CAD build for the part. Positions are in the model's coordinates, mm. Face numbers are marked on the shaded views. A direction names the side the tool comes from. Coordinates: 2 decimals unless noted, no trailing zeros. Loops run counter-clockwise (first coordinate to the right, second up) from the corner with the lowest first, then second, coordinate; pieces in that order, holes last.
1) Saw through at D-D, the plane x = 17. Write the cut outline in (y, z).
2) Pin check, flat tips, straight feed: pin 1 Ø3 at (y, z) = (13.5, 6) entering from -X; pin 2 Ø2 at (x, z) = (45, 4.5) entering from +Y; pin 3 Ø3 at (y, z) = (-2, 4) entering from -X. Stop position of each tip, or through.
3) Two-plate mould, pull along Y, no slides. Class the marked faces 4, 5 and 6: +Y half, -Y half, draft (parallel to the pull), parting line (faces both ways), or undercut.
4) Saw through at B-B, the plane y = -33. Write the cut outline in (x, z), and give its area (3 significant figures).
5) Saw through at C-C, the plane z = 3.25. Give the number of separate pieces and of enclosed holes in the cut face, and give its area (3 significant figures).
6) Wall check: line 1 along Y through (x, z) = (50, 5.25); line 2 along Y through (x, z) = (-13, 6.25); line 3 along X through (y, z) = (12, 1.75). Give the ranges that are in metal, low to high.
7) Saw through at A-A, the plane x = 45. Write the cut outline in (y, z), and give its area (3 significant figures).
8) Which spindle directions (+Z, -Z, +X, -X, +Y, -Y) get a long thin tool onto all of the face, cutting with end or side? Do the marked faces 1, 2 and 3. Say none if no direction does.
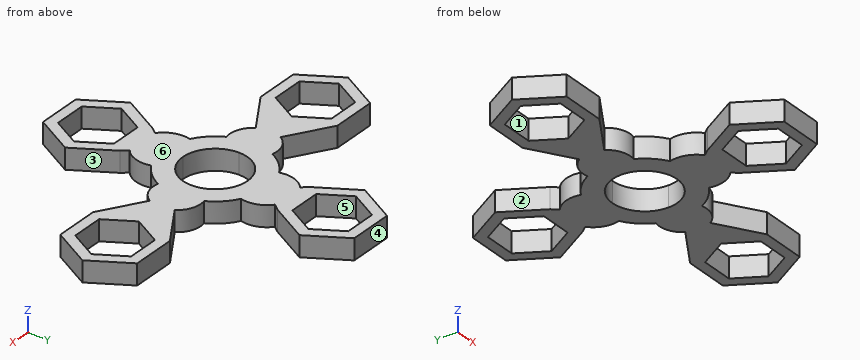
```python
from build123d import *

# Parameters (mm, degrees)
F1_DEPTH = 7


# Not quite as in the source:
# - a feature names something its author has since deleted; it is built from what else it names


with BuildPart() as f1:
    # F0 (on Top) → F1 (new body)
    with BuildSketch(Plane.XY):
        Polygon((-53.4446571767, -12.9903810568), (-38.4446571767, -12.9903810568), (-30.9446571767, 0), (-38.4446571767, 12.9903810568), (-53.4446571767, 12.9903810568), (-60.9446571767, 0), align=None)
        Polygon((-56.8446571767, 0), (-51.3946571767, 9.4396769013), (-40.4946571767, 9.4396769013), (-35.0446571767, 0), (-40.4946571767, -9.4396769013), (-51.3946571767, -9.4396769013), align=None, mode=Mode.SUBTRACT)
        with BuildLine():
            ThreePointArc((0, 10.9), (7.7074639149, 7.7074639149), (10.9, 0))
            Line((10.9, 0), (17.5, 0))
            ThreePointArc((17.5, 0), (17.0367250374, 4), (15.6714285714, 7.78821716))
            ThreePointArc((15.6714285714, 7.78821716), (12.7504247795, 11.9865202599), (8.7403572641, 15.1610077137))
            ThreePointArc((8.7403572641, 15.1610077137), (4.5239565101, 16.9051417473), (0, 17.5))
            Line((0, 17.5), (0, 10.9))
        make_face()
        with BuildLine():
            Line((17.5, 0), (10.9, 0))
            ThreePointArc((10.9, 0), (7.7074639149, -7.7074639149), (0, -10.9))
            Line((0, -10.9), (0, -17.5))
            ThreePointArc((0, -17.5), (4.5925968465, -16.8866235289), (8.8632518819, -15.0894919092))
            ThreePointArc((8.8632518819, -15.0894919092), (12.7990151761, -11.9346223452), (15.6714285714, -7.78821716))
            ThreePointArc((15.6714285714, -7.78821716), (17.0367250374, -4), (17.5, 0))
        make_face()
        with BuildLine():
            ThreePointArc((-10.9, 0), (-7.7074639149, 7.7074639149), (0, 10.9))
            Line((0, 10.9), (0, 17.5))
            ThreePointArc((0, 17.5), (-4.5239565101, 16.9051417473), (-8.7403572641, 15.1610077137))
            ThreePointArc((-8.7403572641, 15.1610077137), (-12.7504247795, 11.9865202599), (-15.6714285714, 7.78821716))
            ThreePointArc((-15.6714285714, 7.78821716), (-17.0367250374, 4), (-17.5, 0))
            Line((-17.5, 0), (-10.9, 0))
        make_face()
        Polygon((-7.5, 26.5479130202), (0, 26.5479130202), (7.5, 26.5479130202), (15, 39.5382940769), (7.5, 52.5286751337), (-7.5, 52.5286751337), (-15, 39.5382940769), align=None)
        Polygon((-10.9, 39.5382940769), (-5.45, 48.9779709782), (5.45, 48.9779709782), (10.9, 39.5382940769), (5.45, 30.0986171757), (-5.45, 30.0986171757), align=None, mode=Mode.SUBTRACT)
        Polygon((30.9, 0), (38.4, -12.9903810568), (53.4, -12.9903810568), (60.9, 0), (53.4, 12.9903810568), (38.4, 12.9903810568), align=None)
        Polygon((40.45, -9.4396769013), (35, 0), (40.45, 9.4396769013), (51.35, 9.4396769013), (56.8, 0), (51.35, -9.4396769013), align=None, mode=Mode.SUBTRACT)
        Polygon((7.5, -26.6851936929), (0, -26.6851936929), (-7.5, -26.6851936929), (-15, -39.6755747497), (-7.5, -52.6659558065), (7.5, -52.6659558065), (15, -39.6755747497), align=None)
        Polygon((-10.9, -39.6755747497), (-5.45, -30.2358978485), (5.45, -30.2358978485), (10.9, -39.6755747497), (5.45, -49.115251651), (-5.45, -49.115251651), align=None, mode=Mode.SUBTRACT)
        with BuildLine():
            Line((0, 26.5479130202), (0, 17.5))
            Line((0, 17.5), (5.7741715282, 24.4658935667))
            ThreePointArc((5.7741715282, 24.4658935667), (3.0690333104, 26.0115077724), (0, 26.5479130202))
        make_face()
        with BuildLine():
            Line((7.5, 26.5479130202), (0, 26.5479130202))
            ThreePointArc((0, 26.5479130202), (3.0690333104, 26.0115077724), (5.7741715282, 24.4658935667))
            Line((5.7741715282, 24.4658935667), (7.5, 26.5479130202))
        make_face()
        with BuildLine():
            ThreePointArc((-5.7741715282, 24.4658935667), (-3.0690333104, 26.0115077724), (0, 26.5479130202))
            Line((0, 26.5479130202), (-7.5, 26.5479130202))
            Line((-7.5, 26.5479130202), (-5.7741715282, 24.4658935667))
        make_face()
        with BuildLine():
            Line((-5.7741715282, 24.4658935667), (0, 17.5))
            Line((0, 17.5), (0, 26.5479130202))
            ThreePointArc((0, 26.5479130202), (-3.0690333104, 26.0115077724), (-5.7741715282, 24.4658935667))
        make_face()
        with BuildLine():
            Line((5.8093756333, -24.6146987236), (0, -17.5))
            Line((0, -17.5), (0, -26.6851936929))
            ThreePointArc((0, -26.6851936929), (3.0836583252, -26.1521000058), (5.8093756333, -24.6146987236))
        make_face()
        with BuildLine():
            ThreePointArc((5.8093756333, -24.6146987236), (3.0836583252, -26.1521000058), (0, -26.6851936929))
            Line((0, -26.6851936929), (7.5, -26.6851936929))
            Line((7.5, -26.6851936929), (5.8093756333, -24.6146987236))
        make_face()
        with BuildLine():
            Line((-7.5, -26.6851936929), (0, -26.6851936929))
            ThreePointArc((0, -26.6851936929), (-3.0836583252, -26.1521000058), (-5.8093756333, -24.6146987236))
            Line((-5.8093756333, -24.6146987236), (-7.5, -26.6851936929))
        make_face()
        with BuildLine():
            Line((0, -26.6851936929), (0, -17.5))
            Line((0, -17.5), (-5.8093756333, -24.6146987236))
            ThreePointArc((-5.8093756333, -24.6146987236), (-3.0836583252, -26.1521000058), (0, -26.6851936929))
        make_face()
        with BuildLine():
            Line((-38.4446571767, -12.9903810568), (-24.2985391386, -4.2166177892))
            ThreePointArc((-24.2985391386, -4.2166177892), (-25.1937738825, -2.1922234023), (-25.5, 0))
            Line((-25.5, 0), (-30.9446571767, 0))
            Line((-30.9446571767, 0), (-38.4446571767, -12.9903810568))
        make_face()
        with BuildLine():
            ThreePointArc((-25.5, 0), (-25.1937738825, 2.1922234023), (-24.2985391386, 4.2166177892))
            Line((-24.2985391386, 4.2166177892), (-38.4446571767, 12.9903810568))
            Line((-38.4446571767, 12.9903810568), (-30.9446571767, 0))
            Line((-30.9446571767, 0), (-25.5, 0))
        make_face()
        with BuildLine():
            ThreePointArc((25.5, 0), (25.1927245669, -2.1959027158), (24.2945028156, -4.2231186922))
            Line((24.2945028156, -4.2231186922), (38.4, -12.9903810568))
            Line((38.4, -12.9903810568), (30.9, 0))
            Line((30.9, 0), (25.5, 0))
        make_face()
        with BuildLine():
            Line((38.4, 12.9903810568), (24.2945028156, 4.2231186922))
            ThreePointArc((24.2945028156, 4.2231186922), (25.1927245669, 2.1959027158), (25.5, 0))
            Line((25.5, 0), (30.9, 0))
            Line((30.9, 0), (38.4, 12.9903810568))
        make_face()
        with BuildLine():
            Line((-24.2985391386, -4.2166177892), (-17.5, 0))
            Line((-17.5, 0), (-22.5, 0))
            Line((-22.5, 0), (-25.5, 0))
            ThreePointArc((-25.5, 0), (-25.1937738825, -2.1922234023), (-24.2985391386, -4.2166177892))
        make_face()
        with BuildLine():
            Line((-22.5, 0), (-17.5, 0))
            Line((-17.5, 0), (-24.2985391386, 4.2166177892))
            ThreePointArc((-24.2985391386, 4.2166177892), (-25.1937738825, 2.1922234023), (-25.5, 0))
            Line((-25.5, 0), (-22.5, 0))
        make_face()
        with BuildLine():
            Line((24.2945028156, 4.2231186922), (17.5, 0))
            Line((17.5, 0), (22.5, 0))
            Line((22.5, 0), (25.5, 0))
            ThreePointArc((25.5, 0), (25.1927245669, 2.1959027158), (24.2945028156, 4.2231186922))
        make_face()
        with BuildLine():
            Line((22.5, 0), (17.5, 0))
            Line((17.5, 0), (24.2945028156, -4.2231186922))
            ThreePointArc((24.2945028156, -4.2231186922), (25.1927245669, -2.1959027158), (25.5, 0))
            Line((25.5, 0), (22.5, 0))
        make_face()
        with BuildLine():
            Line((-5.8093756333, -24.6146987236), (0, -17.5))
            ThreePointArc((0, -17.5), (-4.5925968465, -16.8866235289), (-8.8632518819, -15.0894919092))
            ThreePointArc((-8.8632518819, -15.0894919092), (-8.7466502596, -20.3042632567), (-5.8093756333, -24.6146987236))
        make_face()
        with BuildLine():
            ThreePointArc((8.8632518819, -15.0894919092), (4.5925968465, -16.8866235289), (0, -17.5))
            Line((0, -17.5), (5.8093756333, -24.6146987236))
            ThreePointArc((5.8093756333, -24.6146987236), (8.7466502596, -20.3042632567), (8.8632518819, -15.0894919092))
        make_face()
        with BuildLine():
            Line((24.2945028156, -4.2231186922), (17.5, 0))
            ThreePointArc((17.5, 0), (17.0367250374, -4), (15.6714285714, -7.78821716))
            ThreePointArc((15.6714285714, -7.78821716), (20.5565667679, -7.3930642898), (24.2945028156, -4.2231186922))
        make_face()
        with BuildLine():
            ThreePointArc((15.6714285714, 7.78821716), (17.0367250374, 4), (17.5, 0))
            Line((17.5, 0), (24.2945028156, 4.2231186922))
            ThreePointArc((24.2945028156, 4.2231186922), (20.5565667679, 7.3930642898), (15.6714285714, 7.78821716))
        make_face()
        with BuildLine():
            ThreePointArc((-15.6714285714, -7.78821716), (-17.0367250374, -4), (-17.5, 0))
            Line((-17.5, 0), (-24.2985391386, -4.2166177892))
            ThreePointArc((-24.2985391386, -4.2166177892), (-20.5601021676, -7.3916016346), (-15.6714285714, -7.78821716))
        make_face()
        with BuildLine():
            Line((0, -17.5), (0, -10.9))
            ThreePointArc((0, -10.9), (-7.7074639149, -7.7074639149), (-10.9, 0))
            Line((-10.9, 0), (-17.5, 0))
            ThreePointArc((-17.5, 0), (-17.0367250374, -4), (-15.6714285714, -7.78821716))
            ThreePointArc((-15.6714285714, -7.78821716), (-12.7990151761, -11.9346223452), (-8.8632518819, -15.0894919092))
            ThreePointArc((-8.8632518819, -15.0894919092), (-4.5925968465, -16.8866235289), (0, -17.5))
        make_face()
        with BuildLine():
            Line((-24.2985391386, 4.2166177892), (-17.5, 0))
            ThreePointArc((-17.5, 0), (-17.0367250374, 4), (-15.6714285714, 7.78821716))
            ThreePointArc((-15.6714285714, 7.78821716), (-20.5601021676, 7.3916016346), (-24.2985391386, 4.2166177892))
        make_face()
        with BuildLine():
            ThreePointArc((-8.7403572641, 15.1610077137), (-4.5239565101, 16.9051417473), (0, 17.5))
            Line((0, 17.5), (-5.7741715282, 24.4658935667))
            ThreePointArc((-5.7741715282, 24.4658935667), (-8.6205053042, 20.2480208005), (-8.7403572641, 15.1610077137))
        make_face()
        with BuildLine():
            Line((5.7741715282, 24.4658935667), (0, 17.5))
            ThreePointArc((0, 17.5), (4.5239565101, 16.9051417473), (8.7403572641, 15.1610077137))
            ThreePointArc((8.7403572641, 15.1610077137), (8.6205053042, 20.2480208005), (5.7741715282, 24.4658935667))
        make_face()
    extrude(amount=F1_DEPTH)


solid = f1.part
```
Data:
1. outline: (-7.98, 0) - (7.98, 0) - (7.98, 7) - (-7.98, 7) - close
2. pin 1: stops at x = -54.02
2. pin 2: stops at y = 12.99
2. pin 3: stops at x = -60.66
3. face 4: +Y half
3. face 5: undercut
3. face 6: draft
4. outline: (-11.15, 0) - (-7.05, 0) - (-7.05, 7) - (-11.15, 7) - close; (7.05, 0) - (11.15, 0) - (11.15, 7) - (7.05, 7) - close
4. area: 57.4 mm2
5. separate pieces: 1
5. enclosed holes: 5
5. area: 2,500 mm2
6. line 1: y = -12.99 to -9.44, 9.44 to 12.99
6. line 2: y = -43.14 to -36.21, -11.72 to 11.72, 36.07 to 43
6. line 3: x = -54.02 to -36.85, -12.74 to 12.74, 36.81 to 53.97
7. outline: (-12.99, 0) - (-9.44, 0) - (-9.44, 7) - (-12.99, 7) - close; (9.44, 0) - (12.99, 0) - (12.99, 7) - (9.44, 7) - close
7. area: 49.7 mm2
8. face 1: +Z, -Z
8. face 2: +Z, -Z, -X
8. face 3: +Z, -Z, +X
